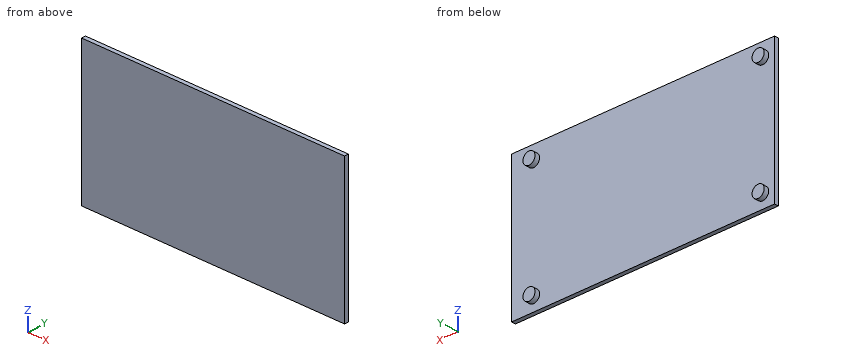
from build123d import *

# Parameters (mm, degrees)
SKETCH1_W           = 95.6
SKETCH1_H           = 51.6
BOSS_EXTRUDE1_DEPTH = 1.5
SKETCH2_R           = 2.2
BOSS_EXTRUDE2_DEPTH = 1.8


with BuildPart() as part:
    # Sketch1 → Boss-Extrude1 (new body)
    with BuildSketch(Plane.XZ.offset(1)):
        with Locations((0, 36)):
            Rectangle(SKETCH1_W, SKETCH1_H)
    extrude(amount=BOSS_EXTRUDE1_DEPTH)

    # Sketch2 → Boss-Extrude2 (add)
    with BuildSketch(Plane(origin=(0, -1, 0), x_dir=(1, 0, 0), z_dir=(0, 1, 0))):
        with Locations((-43.453932042, -56.8)):
            Circle(SKETCH2_R)
        with Locations((-43.453932042, -15)):
            Circle(SKETCH2_R)
        with Locations((39.832771039, -15)):
            Circle(SKETCH2_R)
        with Locations((39.832771039, -56.8)):
            Circle(SKETCH2_R)
    extrude(amount=BOSS_EXTRUDE2_DEPTH)


solid = part.part
The listing builds one solid part. Answer for the finished solid, in the listing's coordinates (mm). Round coordinates to 2 decimals unless told otherwise and drop trailing zeros. Loops run counter-clockwise (first coordinate to the right, second up) from the corner with the lowest first, then second, coordinate; pieces in that order, holes last. Notation, with made-up numbers: M 77.5,31 L 111.5,31 A23 cw 111.5,63 Z; hole C 26.25,-23 d3. An arc over 180 degrees is marked long. Write each question's results on one line, items separated by ' | '. Start each with the question number.
1) Find section C-C on x = -12. Write down the section's boundary in (y, z), plus the area to 3 significant figures.
2) Straight lines are drawn through the part: probe 1 along Y at (x, z) = (29, 18); probe 2 along X at (y, z) = (-0.65, 14.5); probe 3 along X at (y, z) = (-0.95, 13.5). For each, find the intervals that lie inside material, in ascending order.
3) This flat-tipped pin is pushed along its axis until it touches: pin 1 (10 mm diameter, centred on x = -14, z = 41.5, fed in from +Y). Where does it stop, or does it pass through?
4) Find section A-A on z = 15. Write down the section's boundary in (x, y), plus the area to 3 significant figures.
5) Find section B-B on y = -0.45. Write down the section's boundary in (x, z), plus the area to 3 significant figures.
6) Find section D-D on z = 37.5. Write down the section's boundary in (x, y), plus the area to 3 significant figures.
Final values:
1) outline: M -2.5,10.2 L -1,10.2 L -1,61.8 L -2.5,61.8 Z | area: 77.4 mm²
2) probe 1: -2.5 to -1 | probe 2: -45.6 to -41.31, 37.69 to 41.98 | probe 3: -45.06 to -41.84, 38.22 to 41.44
3) pin 1: y = -1
4) outline: M -47.8,-2.5 L 47.8,-2.5 L 47.8,-1 L 42.03,-1 L 42.03,0.8 L 37.63,0.8 L 37.63,-1 L -41.25,-1 L -41.25,0.8 L -45.65,0.8 L -45.65,-1 L -47.8,-1 Z | area: 159 mm²
5) outline: C -43.45,15 d4.4; C -43.45,56.8 d4.4; C 39.83,15 d4.4; C 39.83,56.8 d4.4 | area: 60.8 mm²
6) outline: M -47.8,-2.5 L 47.8,-2.5 L 47.8,-1 L -47.8,-1 Z | area: 143 mm²
